Could you check a few things on this model? Use its own coordinates, in mm. A direction names the side the tool comes from. Give positions to 0.01 mm unless a question says otherwise; leave off trailing zeros. Loops run counter-clockwise (first coordinate to the right, second up) from the corner with the lowest first, then second, coordinate; pieces in that order, holes last. Notation, with made-up numbers: (2, -33) - (57, -33) arc R20 cw to (57, -28) - close; hole circle Ø1 at (53, 69). An arc over 180 degrees is marked (long way). One line per item, written item: value. Start each with the question number.
Q1. For faces 5 (the face through (40, 13, 6)), 6 (the face through (4.336, 37.535, 303.476)), 7 (the face through (-40, 14, 6)), 8 (the face through (-1, -5, 341)), 9 (the face through (0, 35, 5)), which set-ups out of +Z, -Z, +X, -X, +Y, -Y let a thin tool reach every point of the face, with its end or its side?
Q2. If we mould it in two halves opening along Y, with no side actions, what happens to faces 1 (the face through (-1, 0, 341)), 2 (the face through (-3, 36, 379)), 3 (the face through (-1, -5, -341)), 4 (the face through (-35, 13, 6))? For each: released by +Y, released by -Y, zero draft, split by the parting line, or undercut.
Q3. I'm going to push flat-ended pins straight in: P1, Ø2.5, axis at x = 2.5, y = 38.5, coming from the +Z side; P2, Ø5, axis at y = 16, z = 289.5, coming from the +X side; P3, Ø5.5, axis at x = -37, y = 12, coming from the -Z side. Where does each tip first touch, or does it pass through?
Q4. If I drill on line 1 (Z direction, x = 0, y = -1.9); line 2 (X direction, y = 27.5, z = 328.5); line 3 (Z direction, x = 0, y = 36.45), over which ranges is the centre line in solid material (lowest first)? Write a range as from..to.
Q5. I want a section at A-A (z = -49). Please give me the cut outline in (x, y).
```python
from build123d import *

# Parameters (mm, degrees)
F1_DEPTH  = 395
F2_R      = 20
F3_DEPTH  = 40.001
F4_W      = 5
F4_H      = 120
F5_DEPTH  = 5
F6_SIZE   = 5
F7_R      = 6.5
F8_DEPTH  = 45.001
F11_DEPTH = 85.001


with BuildPart() as f1:
    # F0 (on Top) → F1 (new body, symmetric)
    with BuildSketch(Plane.XY):
        with BuildLine():
            Line((27, 40), (-27, 40))
            ThreePointArc((-27, 40), (-36.1923881554, 36.1923881554), (-40, 27))
            Line((-40, 27), (-40, 0))
            Line((-40, 0), (-35, 0))
            Line((-35, 0), (-35, 27))
            ThreePointArc((-35, 27), (-32.6568542495, 32.6568542495), (-27, 35))
            Line((-27, 35), (27, 35))
            ThreePointArc((27, 35), (32.6568542495, 32.6568542495), (35, 27))
            Line((35, 27), (35, 0))
            Line((35, 0), (40, 0))
            Line((40, 0), (40, 27))
            ThreePointArc((40, 27), (36.1923881554, 36.1923881554), (27, 40))
        make_face()
    extrude(amount=F1_DEPTH, both=True)

    # F2 (on face) → F3 (cut, through all)
    with BuildSketch(Plane(origin=(0, 40, 0), x_dir=(-1, 0, 0), z_dir=(0, 1, 0))):
        with Locations((0, 323)):
            Circle(F2_R)
        with BuildLine():
            Line((-7.5, 127.5), (7.5, 127.5))
            ThreePointArc((7.5, 127.5), (13, 133), (7.5, 138.5))
            Line((7.5, 138.5), (-7.5, 138.5))
            ThreePointArc((-7.5, 138.5), (-13, 133), (-7.5, 127.5))
        make_face()
        with BuildLine():
            ThreePointArc((-7.5, -127.5), (-13, -133), (-7.5, -138.5))
            Line((-7.5, -138.5), (7.5, -138.5))
            ThreePointArc((7.5, -138.5), (13, -133), (7.5, -127.5))
            Line((7.5, -127.5), (-7.5, -127.5))
        make_face()
        with Locations((0, -323)):
            Circle(F2_R)
    extrude(amount=-F3_DEPTH, mode=Mode.SUBTRACT)

    # F4 (on face) → F5 (join)
    with BuildSketch(Plane.XZ):
        Polygon((45, 405), (-45, 405), (-45, 275), (-40, 275), (-40, 395), (-35, 395), (-35, 275), (45, 275), align=None)
        with Locations((-37.5, 335)):
            Rectangle(F4_W, F4_H)
    extrude(amount=F5_DEPTH)

    # F6
    f6_edges = [f1.edges().sort_by_distance(p)[0] for p in [
        (45, -2.5, 275),
        (-45, -2.5, 275),
        (-45, -2.5, 405),
        (45, -2.5, 405),
    ]]
    chamfer(f6_edges, length=F6_SIZE)

    # F7 (on face) → F8 (cut, through all)
    with BuildSketch(Plane.XZ.offset(5)):
        with Locations((0, 323)):
            Circle(F7_R)
    extrude(amount=-F8_DEPTH, mode=Mode.SUBTRACT)

    # F9: F1 across plane


with BuildPart() as f1_1:
    add(f1.part)
    add(f1.part.mirror(Plane.XY))

    # F10 (on face) → F11 (cut, through all)
    with BuildSketch(Plane.YZ.offset(40)):
        Polygon((27, 388), (27, 395), (20, 395), align=None)
        Polygon((40, 375), (40, 395), (27, 395), (27, 388), align=None)
        Polygon((27, -395), (27, -388), (20, -395), align=None)
        Polygon((40, -375), (27, -388), (27, -395), (40, -395), align=None)
    extrude(amount=-F11_DEPTH, mode=Mode.SUBTRACT)


solid = f1_1.part
```
Worked answers:
1. face 5: +Z, -Z, +X, +Y
1. face 6: +Y
1. face 7: +Z, -Z, -X, +Y
1. face 8: +Z, -Z, +X, -X, -Y
1. face 9: +Z, -Z
2. face 1: undercut
2. face 2: released by +Y
2. face 3: released by -Y
2. face 4: undercut
3. P1: stops at z = 377.75
3. P2: stops at x = 40
3. P3: stops at z = -395
4. line 1: z = -405..-329.5, -316.5..-275, 275..316.5, 329.5..405
4. line 2: x = -39.99..-34.98, 34.98..39.99
4. line 3: z = -378.55..-343, -303..-138.5, -127.5..127.5, 138.5..303, 343..378.55
5. outline: (-40, 0) - (-35, 0) - (-35, 27) arc R8 cw to (-27, 35) - (27, 35) arc R8 cw to (35, 27) - (35, 0) - (40, 0) - (40, 27) arc R13 ccw to (27, 40) - (-27, 40) arc R13 ccw to (-40, 27) - close
